from build123d import *

# Parameters (mm, degrees)
ESQUISSE1_R        = 4
ESQUISSE1_R_2      = 1.15
ESQUISSE1_R_3      = 1.5
BOSS_EXTRU_1_DEPTH = 5
CONG_1_R           = 10
CONG_2_R           = 20


with BuildPart() as part:
    # Esquisse1 → Boss.-Extru.1 (new body)
    with BuildSketch(Plane.XY):
        Polygon((-21.5, 0), (-25, 0), (-25, -5), (-30, -5), (-30, 0), (-35, 0), (-35, 20), (-45, 60), (-45, 100), (14.886620542, 100), (90, 210), (90, 250), (117.313956166, 250), (150, 250), (150, 255), (155, 255), (155, 250), (158.5, 250), (158.5, 247), (157.4, 247), (157.4, 244.7), (158.5, 244.7), (158.5, 240), (161.5, 240), (161.5, 244.7), (162.6, 244.7), (162.6, 247), (161.5, 247), (161.5, 250), (165, 250), (165, 255), (170, 255), (170, 250), (210, 250), (210, 210), (195, 210), (195, 0), (190, 0), (190, -5), (185, -5), (185, 0), (181.5, 0), (181.5, 3), (182.6, 3), (182.6, 5.3), (181.5, 5.3), (181.5, 10), (178.5, 10), (178.5, 5.3), (177.4, 5.3), (177.4, 3), (178.5, 3), (178.5, 0), (175, 0), (175, -5), (170, -5), (170, 0), (165, 0), (165, 25), (52.470534613, 101.840622125), (0, 25), (0, 0), (-10, 0), (-10, -5), (-15, -5), (-15, 0), (-18.5, 0), (-18.5, 3), (-17.4, 3), (-17.4, 5.3), (-18.5, 5.3), (-18.5, 10), (-21.5, 10), (-21.5, 5.3), (-22.6, 5.3), (-22.6, 3), (-21.5, 3), align=None)
        with Locations((135, 230)):
            Circle(ESQUISSE1_R, mode=Mode.SUBTRACT)
        with Locations((195, 230)):
            Circle(ESQUISSE1_R, mode=Mode.SUBTRACT)
        with Locations((105, 230)):
            Circle(ESQUISSE1_R, mode=Mode.SUBTRACT)
        with Locations((86.729297438, 178.610587107)):
            Circle(ESQUISSE1_R_2, mode=Mode.SUBTRACT)
        with Locations((180.729297438, 96.610587107)):
            Circle(ESQUISSE1_R_2, mode=Mode.SUBTRACT)
        with Locations((86.729297438, 96.610587107)):
            Circle(ESQUISSE1_R_2, mode=Mode.SUBTRACT)
        with Locations((180.729297438, 178.610587107)):
            Circle(ESQUISSE1_R_2, mode=Mode.SUBTRACT)
        with Locations((-24.543125869, 83.023041686)):
            Circle(ESQUISSE1_R_3, mode=Mode.SUBTRACT)
        Polygon((165, 210), (126.32704727, 210), (69.388067414, 126.61555066), (165, 61.32704727), align=None, mode=Mode.SUBTRACT)
        Polygon((-29.672175025, 80.799788495), (-32.886113073, 76.969566279), (-29.055890858, 73.755628231), (-25.841952809, 77.585850447), align=None, mode=Mode.SUBTRACT)
        Polygon((-23.244298928, 88.460232926), (-20.03036088, 92.290455142), (-16.200138664, 89.076517093), (-19.414076712, 85.246294878), align=None, mode=Mode.SUBTRACT)
    extrude(amount=BOSS_EXTRU_1_DEPTH)

    # Congé1
    cong_1_edges = [part.edges().sort_by_distance(p)[0] for p in [
        (-35, 20, 2.5),
        (-45, 60, 2.5),
        (-45, 100, 2.5),
        (14.886620542, 100, 2.5),
        (90, 210, 2.5),
        (195, 210, 2.5),
        (165, 25, 2.5),
        (52.470534613, 101.840622125, 2.5),
        (0, 25, 2.5),
        (126.32704727, 210, 2.5),
        (69.388067414, 126.61555066, 2.5),
        (165, 61.32704727, 2.5),
        (165, 210, 2.5),
    ]]
    fillet(cong_1_edges, radius=CONG_1_R)

    # Congé2
    cong_2_edges = [part.edges().sort_by_distance(p)[0] for p in [
        (90, 250, 2.5),
        (210, 250, 2.5),
        (210, 210, 2.5),
    ]]
    fillet(cong_2_edges, radius=CONG_2_R)


solid = part.part
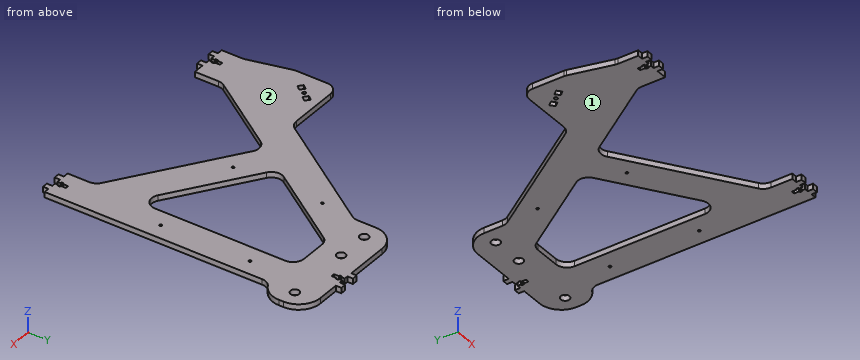
Can you work these out from the model? Positions are in its coordinate system, mm. Face numbers are marked on the shaded views. Coordinates: 2 decimals unless noted, no trailing zeros. Write each loop counter-clockwise with the first axis right and the second up, starting at its lowest first coordinate (ties: lowest second). Pieces come first, ordered by that corner, then holes. Notation, with made-up numbers: (-28, 17.5) -> (2, 17.5) arc R6 ccw to (2, 27.5) -> close; hole circle Ø10 at (5.25, 3). An arc over 180 degrees is marked (long way). Write each question's results on one line, items separated by ' | '. Start each with the question number.
Item 1: Please list where these lines run through material, in increasing order: probe 1 along Y at (x, z) = (133, 3.2); probe 2 along X at (y, z) = (86, 4.65); probe 3 along Y at (x, z) = (-9, 1.75).
Item 2: If we section it at C-C, the plane y = 51.5: Write out the boundary of the cut face in (x, z) (1 decimal), and give its area (3 significant figures).
Item 3: I'm going to push flat-ended pins straight in: P1, Ø0.6, axis at x = -22, z = 3.5, coming from the +Y side; P2, Ø2.5, axis at y = 131, z = 1.5, coming from the -X side; P3, Ø0.9, axis at x = 162, z = 1.5, coming from the -Y side; P4, Ø10.5, axis at x = 105, y = 230, coming from the -Z side. Where does each tip first touch, or does it pass through?
Item 4: If we section it at B-B, the plane x = 135: Write out the boundary of the cut face in (y, z).
Item 5: If we section it at D-D, the plane z = 1.2: Count the separate pieces of the cut face and the enclosed holes in it, and give its area (3 significant figures).
Item 6: Thinking about a two-plate mould opening in Z: for the marked faces 1 and 2, which applies, released by +Z, released by -Z, zero draft, split by the parting line, or undercut?
Item 7: If we section it at A-A, the plane y = 170.5: Write out the boundary of the cut face in (x, z).
Answer block:
1) probe 1: 46.85 to 83.18, 210 to 226.54, 233.46 to 250 | probe 2: -45 to -20.31, -18.78 to 41.65, 75.67 to 128.87, 165 to 195 | probe 3: 0 to 100
2) outline: (-42.9, 0) -> (18.1, 0) -> (18.1, 5) -> (-42.9, 5) -> close; (126.2, 0) -> (195, 0) -> (195, 5) -> (126.2, 5) -> close | area: 649 mm²
3) P1: y = 100 | P2: x = 35.2 | P3: y = 26.39 | P4: z = 0
4) outline: (45.49, 0) -> (81.81, 0) -> (81.81, 5) -> (45.49, 5) -> close; (210, 0) -> (226, 0) -> (226, 5) -> (210, 5) -> close; (234, 0) -> (250, 0) -> (250, 5) -> (234, 5) -> close
5) separate pieces: 1 | enclosed holes: 11 | area: 24,700 mm²
6) face 1: released by -Z | face 2: released by +Z
7) outline: (63.03, 0) -> (99.35, 0) -> (99.35, 5) -> (63.03, 5) -> close; (165, 0) -> (195, 0) -> (195, 5) -> (165, 5) -> close
